```python
from build123d import *

# Parameters (mm, degrees)
F0_W     = 65.131832
F0_H     = 64.514473
F1_DEPTH = 10
F3_DEPTH = 43
F4_DEPTH = 21


with BuildPart() as f1:
    # F0 (on Front) → F1 (new body)
    with BuildSketch(Plane.XZ):
        with Locations((1.729728, -11.223505)):
            Rectangle(F0_W, F0_H)
        with BuildLine():
            ThreePointArc((8.682307, 11.441543), (8.729724, 10.635549), (8.684016, 9.829457))
            Line((8.684016, 9.829457), (8.729724, -33.286821))
            ThreePointArc((8.729724, -33.286821), (1.936423, -40.29119), (-5.258499, -33.700043))
            ThreePointArc((-5.258499, -33.700043), (-5.270272, -33.294242), (-5.258499, -32.888441))
            Line((-5.258499, -32.888441), (-5.258499, 10.222327))
            ThreePointArc((-5.258499, 10.222327), (-5.270272, 10.628129), (-5.258499, 11.03393))
            ThreePointArc((-5.258499, 11.03393), (1.525143, 17.625138), (8.682307, 11.441543))
        make_face(mode=Mode.SUBTRACT)
    extrude(amount=F1_DEPTH)

    # F2 (on Top) → F3 (join)
    with BuildSketch(Plane.XY):
        Polygon((-29.885342, 0), (-24.503149, 0), (-24.503149, 20.254048), (-17.98786, 20.254048), (-17.98786, 24.219874), (-36.117356, 24.219874), (-36.117356, 20.254048), (-29.885342, 20.254048), align=None)
        Polygon((29.318795, 0), (34.417719, 0), (34.417719, 20.254048), (40.649734, 20.254048), (40.649734, 24.219874), (23.653327, 24.219874), (23.653327, 20.254048), (29.318795, 20.254048), align=None)
    extrude(amount=-F3_DEPTH)

    # F3_face (on face) → F4 (join)
    with BuildSketch(Plane(origin=(31.980128, 14.909508, 0), x_dir=(1, 0, 0), z_dir=(0, 0, 1))):
        Polygon((-2.661333, -14.909508), (2.315516, -14.909508), (2.437591, -14.909508), (2.437591, 5.34454), (8.669607, 5.34454), (8.669607, 9.310366), (-8.326801, 9.310366), (-8.326801, 5.34454), (-2.661333, 5.34454), align=None)
        Polygon((-61.86547, -14.909508), (-56.483277, -14.909508), (-56.483277, 5.34454), (-49.967988, 5.34454), (-49.967988, 9.310366), (-68.097484, 9.310366), (-68.097484, 5.34454), (-61.86547, 5.34454), align=None)
    extrude(amount=F4_DEPTH)


solid = f1.part
```
Geometry check sheet. Reference: the model listing, model coordinates, mm. A direction names the side the tool comes from. Coordinates: 2 decimals unless noted, no trailing zeros. Write each loop counter-clockwise with the first axis right and the second up, starting at its lowest first coordinate (ties: lowest second). Pieces come first, ordered by that corner, then holes. Notation, with made-up numbers: (20.25, -2.5) -> (72.25, -2.5) arc R17 ccw to (72.25, 27.5) -> close; hole circle Ø7 at (-1.5, 34). An arc over 180 degrees is marked (long way). Use CSV: the item, a comma, the result in double quotes. Start each with the question number.
Item 1: Cross-section at B-B, the plane x = -23.5. Record the cut outline in (y, z).
Item 2: Cross-section at D-D, the plane z = -3.5. Record the cut outline in (x, y).
Item 3: Mould release check, pull along X, two halves, no side actions. Record for faces 1 (the flat face through (-29.885, 10, -11)), 2 (the flat face through (26, 20.254, -11)), 3 (the flat face through (-27, 15, 21)), 4 (the flat face through (29.319, 10, -11)): released by +X, released by -X, zero draft, split by the parting line, or undercut.
Item 4: Cross-section at C-C, the plane z = -30. Record the cut outline in (x, y), plus the area to 3 significant figures.
Item 5: Thickness scan on line 1 (X direction, y = 3.5, z = -36.5); line 2 (X direction, y = 21, z = 16.5); line 3 (Y direction, x = 25.5, z = 14). Record the ranges inside material, lowest first.
Item 6: Cross-section at A-A, the plane y = 2. Record the cut outline in (x, z), plus the area to 3 significant figures.
Item 7: Depth check by flat-ended pin: pin 1 Ø3 at (y, z) = (13, -8) entering from -X; pin 2 Ø1.9 at (x, z) = (37, -0.5) entering from -Y; pin 3 Ø5 at (y, z) = (2, -11) entering from -X. Enter the tip coordinate at first touch or a pass-through.
Item 8: Set-up check for faces 5 (the flat face through (34.296, -5, -12)), 6 (the cylindrical face through (1.38, -4.93, 17.62)), 7 (the flat face through (-21, 20.254, -11)), 8 (the flat face through (-27, 24.22, -11)): record each of +Z, -Z, +X, -X, +Y, -Y from which the full face is reachable in a straight line by a thin tool's end or side.
Answers:
1,outline,"(-10, -43.48) -> (0, -43.48) -> (0, 21.03) -> (-10, 21.03) -> close; (20.25, -43) -> (24.22, -43) -> (24.22, 21) -> (20.25, 21) -> close"
2,outline,"(-36.12, 20.25) -> (-29.89, 20.25) -> (-29.89, 0) -> (-30.84, 0) -> (-30.84, -10) -> (-5.26, -10) -> (-5.26, 0) -> (-24.5, 0) -> (-24.5, 20.25) -> (-17.99, 20.25) -> (-17.99, 24.22) -> (-36.12, 24.22) -> close; (8.7, -10) -> (34.3, -10) -> (34.3, 0) -> (34.42, 0) -> (34.42, 20.25) -> (40.65, 20.25) -> (40.65, 24.22) -> (23.65, 24.22) -> (23.65, 20.25) -> (29.32, 20.25) -> (29.32, 0) -> (8.7, 0) -> close"
3,face 1,"released by -X"
3,face 2,"undercut"
3,face 3,"zero draft"
3,face 4,"undercut"
4,outline,"(-36.12, 20.25) -> (-29.89, 20.25) -> (-29.89, 0) -> (-30.84, 0) -> (-30.84, -10) -> (-5.26, -10) -> (-5.26, 0) -> (-24.5, 0) -> (-24.5, 20.25) -> (-17.99, 20.25) -> (-17.99, 24.22) -> (-36.12, 24.22) -> close; (8.73, -10) -> (34.3, -10) -> (34.3, 0) -> (34.42, 0) -> (34.42, 20.25) -> (40.65, 20.25) -> (40.65, 24.22) -> (23.65, 24.22) -> (23.65, 20.25) -> (29.32, 20.25) -> (29.32, 0) -> (8.73, 0) -> close"
4,area,"863 mm^2"
5,line 1,"-29.89 to -24.5, 29.32 to 34.42"
5,line 2,"-36.12 to -17.99, 23.65 to 40.65"
5,line 3,"-10 to 0, 20.25 to 24.22"
6,outline,"(-29.89, -43) -> (-24.5, -43) -> (-24.5, 21) -> (-29.89, 21) -> close; (29.32, -43) -> (34.42, -43) -> (34.42, 21) -> (29.32, 21) -> close"
6,area,"671 mm^2"
7,pin 1,"x = -29.89"
7,pin 2,"y = 20.25"
7,pin 3,"x = -30.84"
8,face 5,"+Z, -Z, +X, -Y"
8,face 6,"+Y, -Y"
8,face 7,"+Z, -Z"
8,face 8,"+Z, -Z, +X, -X, +Y"
